from build123d import *

# Parameters (mm, degrees)
F2_W     = 1
F2_H     = 9.471692
F3_DEPTH = 2


with BuildPart() as f1:
    # F0 (on Front) → F1 (revolve)
    with BuildSketch(Plane.XZ):
        Polygon((-3, 0), (0, 0), (0, 20), (-2.5, 22.5), (-3, 22.5), align=None)
    revolve(axis=Axis((0, 0, 10), (0, 0, -1)))

    # F2 (on face) → F3 (cut)
    with BuildSketch(Plane(origin=(0, 0, 0), x_dir=(1, 0, 0), z_dir=(0, 0, -1))):
        Rectangle(F2_W, F2_H)
    extrude(amount=-F3_DEPTH, mode=Mode.SUBTRACT)


solid = f1.part
Geometry: final body of the model. Coordinates: model frame, mm. A direction names the side the tool comes from. Round coordinates to 2 decimals unless told otherwise and drop trailing zeros. Order: outer loops, then holes, each group sorted by start corner. A loop starts at its lowest first (then second) coordinate and runs counter-clockwise, first axis right, second up.
Q1. Mould query, pull axis Y, two halves, no side actions, for faces 1 (the face through (0.65, -2.93, 11.09)), 2 (the face through (-1, 0, 0)), 3 (the face through (0, -1, 21)). Classes: released by +Y, released by -Y, zero draft, split by the parting line, or undercut.
Result sheet:
face 1: split by the parting line
face 2: zero draft
face 3: undercut
Q2. Section A-A, the plane z = 16.75. Output: boundary loops of the cut face in (x, y).
Result sheet:
outline: circle Ø6 at (0, 0)
Q3. Access query for faces 4 (the face through (-2, 2, 22.5)), 5 (the face through (0.5, 0, 1)). Directions: +Z, -Z, +X, -X, +Y, -Y. A direction counts if a zero-diameter tool reaches every point of the face in a straight line with its end or side. Return the directions, or none.
Result sheet:
face 4: +Z, +X, -X, +Y, -Y
face 5: -Z, +Y, -Y
Q4. Pin query (flat end, axial travel): pin 1 (1 mm diameter, centred on x = -1.5, z = 19, fed in from -Y); pin 2 (0.6 mm diameter, centred on y = 1.5, z = 1.5, fed in from -X); pin 3 (1.5 mm diameter, centred on y = -1, z = 14.5, fed in from -X). Return the tip coordinate at first contact, or that it passes through.
Result sheet:
pin 1: stops at y = -2.83
pin 2: stops at x = -2.75
pin 3: stops at x = -2.99
Q5. Material intervals for probe 1 along X at (y, z) = (-1.75, 1.75); probe 2 along Y at (x, z) = (-1.65, 2); probe 3 along X at (y, z) = (-0.5, 6), sorted ascending.
Result sheet:
probe 1: x = -2.44 to -0.5, 0.5 to 2.44
probe 2: y = -2.51 to 2.51
probe 3: x = -2.96 to 2.96
